Work out the finished part from the listing and answer in its coordinate system (mm). A direction names the side the tool comes from. Round coordinates to 2 decimals unless told otherwise and drop trailing zeros. Order: outer loops, then holes, each group sorted by start corner. A loop starts at its lowest first (then second) coordinate and runs counter-clockwise, first axis right, second up. Notation, with made-up numbers: (-30, 19.25) - (-15, 19.25) arc R10 cw to (-15, 38.25) - close; hole circle Ø2 at (49.5, 71). An arc over 180 degrees is marked (long way). Answer in a Markdown table with one row per item.
from build123d import *

# Parameters (mm, degrees)
SKETCH8_W           = 131.76
SKETCH8_H           = 95.69
SKETCH8_R           = 3.43
SKETCH8_W_2         = 73.4
SKETCH8_H_2         = 33.99
BOSS_EXTRUDE4_DEPTH = 40
SKETCH9_R           = 8
CUT_EXTRUDE2_DEPTH  = 8
SKETCH12_W          = 9.12
SKETCH12_H          = 95.69
BOSS_EXTRUDE5_DEPTH = 40
SKETCH13_W          = 150
SKETCH13_H          = 50.05
BOSS_EXTRUDE6_DEPTH = 26.38
SKETCH14_R          = 3.05
CUT_EXTRUDE3_DEPTH  = 3.05


with BuildPart() as part:
    # Sketch8 → Boss-Extrude4 (new body)
    with BuildSketch(Plane(origin=(0, 0, 0), x_dir=(1, 0, 0), z_dir=(0, 1, 0))):
        with Locations((-55.88, 37.845)):
            Rectangle(SKETCH8_W, SKETCH8_H)
        with Locations((-100.58, 12.85)):
            Circle(SKETCH8_R, mode=Mode.SUBTRACT)
        with Locations((-100.58, 62.84)):
            Circle(SKETCH8_R, mode=Mode.SUBTRACT)
        with Locations((-11.18, 62.84)):
            Circle(SKETCH8_R, mode=Mode.SUBTRACT)
        with Locations((-11.18, 12.85)):
            Circle(SKETCH8_R, mode=Mode.SUBTRACT)
        with Locations((-55.88, 37.845)):
            Rectangle(SKETCH8_W_2, SKETCH8_H_2, mode=Mode.SUBTRACT)
    extrude(amount=BOSS_EXTRUDE4_DEPTH)

    # Sketch9 → Cut-Extrude2 (cut)
    with BuildSketch(Plane.XZ):
        with Locations((-100.58, -12.85)):
            Circle(SKETCH9_R)
        with Locations((-11.18, -12.85)):
            Circle(SKETCH9_R)
        with Locations((-11.18, -62.84)):
            Circle(SKETCH9_R)
        with Locations((-100.58, -62.84)):
            Circle(SKETCH9_R)
    extrude(amount=-CUT_EXTRUDE2_DEPTH, mode=Mode.SUBTRACT)

    # Sketch12 → Boss-Extrude5 (add)
    with BuildSketch(Plane.XZ):
        with Locations((-126.32, -37.845)):
            Rectangle(SKETCH12_W, SKETCH12_H)
        with Locations((14.56, -37.845)):
            Rectangle(SKETCH12_W, SKETCH12_H)
    extrude(amount=-BOSS_EXTRUDE5_DEPTH)

    # Sketch13 → Boss-Extrude6 (add)
    with BuildSketch(Plane.XZ):
        with Locations((-55.88, 35.025)):
            Rectangle(SKETCH13_W, SKETCH13_H)
    extrude(amount=-BOSS_EXTRUDE6_DEPTH)

    # Sketch14 → Cut-Extrude3 (cut)
    with BuildSketch(Plane(origin=(0, 26.38, 0), x_dir=(1, 0, 0), z_dir=(0, 1, 0))):
        with Locations((-105.88, -22.5125)):
            Circle(SKETCH14_R)
        with Locations((-105.88, -47.5375)):
            Circle(SKETCH14_R)
        with BuildLine():
            ThreePointArc((-77.83, -35.025), (-80.88, -31.975), (-83.93, -35.025))
            Line((-83.93, -35.025), (-77.83, -35.025))
        make_face()
        with BuildLine():
            Line((-77.83, -35.025), (-83.93, -35.025))
            ThreePointArc((-83.93, -35.025), (-80.88, -38.075), (-77.83, -35.025))
        make_face()
        with BuildLine():
            ThreePointArc((-52.83, -22.5125), (-53.723324317, -20.355824317), (-55.88, -19.4625))
            Line((-55.88, -19.4625), (-55.88, -25.5625))
            ThreePointArc((-55.88, -25.5625), (-53.723324317, -24.669175683), (-52.83, -22.5125))
        make_face()
        with BuildLine():
            Line((-55.88, -25.5625), (-55.88, -19.4625))
            ThreePointArc((-55.88, -19.4625), (-58.93, -22.5125), (-55.88, -25.5625))
        make_face()
        with BuildLine():
            ThreePointArc((-55.88, -44.4875), (-58.93, -47.5375), (-55.88, -50.5875))
            Line((-55.88, -50.5875), (-55.88, -44.4875))
        make_face()
        with BuildLine():
            Line((-55.88, -44.4875), (-55.88, -50.5875))
            ThreePointArc((-55.88, -50.5875), (-53.723324317, -49.694175683), (-52.83, -47.5375))
            ThreePointArc((-52.83, -47.5375), (-53.723324317, -45.380824317), (-55.88, -44.4875))
        make_face()
        with BuildLine():
            ThreePointArc((-33.93, -35.025), (-33.036675683, -37.181675683), (-30.88, -38.075))
            Line((-30.88, -38.075), (-30.88, -35.025))
            Line((-30.88, -35.025), (-33.93, -35.025))
        make_face()
        with BuildLine():
            Line((-30.88, -35.025), (-30.88, -38.075))
            ThreePointArc((-30.88, -38.075), (-28.723324317, -37.181675683), (-27.83, -35.025))
            Line((-27.83, -35.025), (-30.88, -35.025))
        make_face()
        with BuildLine():
            ThreePointArc((-27.83, -35.025), (-28.723324317, -32.868324317), (-30.88, -31.975))
            Line((-30.88, -31.975), (-30.88, -35.025))
            Line((-30.88, -35.025), (-27.83, -35.025))
        make_face()
        with BuildLine():
            Line((-30.88, -35.025), (-30.88, -31.975))
            ThreePointArc((-30.88, -31.975), (-33.036675683, -32.868324317), (-33.93, -35.025))
            Line((-33.93, -35.025), (-30.88, -35.025))
        make_face()
        with BuildLine():
            ThreePointArc((-2.83, -22.5125), (-3.723324317, -20.355824317), (-5.88, -19.4625))
            Line((-5.88, -19.4625), (-5.88, -25.5625))
            ThreePointArc((-5.88, -25.5625), (-3.723324317, -24.669175683), (-2.83, -22.5125))
        make_face()
        with BuildLine():
            Line((-5.88, -25.5625), (-5.88, -19.4625))
            ThreePointArc((-5.88, -19.4625), (-8.93, -22.5125), (-5.88, -25.5625))
        make_face()
        with BuildLine():
            ThreePointArc((-5.88, -44.4875), (-8.93, -47.5375), (-5.88, -50.5875))
            Line((-5.88, -50.5875), (-5.88, -44.4875))
        make_face()
        with BuildLine():
            Line((-5.88, -44.4875), (-5.88, -50.5875))
            ThreePointArc((-5.88, -50.5875), (-3.723324317, -49.694175683), (-2.83, -47.5375))
            ThreePointArc((-2.83, -47.5375), (-3.723324317, -45.380824317), (-5.88, -44.4875))
        make_face()
    extrude(amount=-CUT_EXTRUDE3_DEPTH, mode=Mode.SUBTRACT)


solid = part.part
1) The mould has two halves that part along X. Classify faces 1 (the face through (-57, 13, 60.05)), 2 (the face through (-6, 23.33, 22)): released by +X, released by -X, zero draft, split by the parting line, or undercut.
Filled in:
| item | result |
|---|---|
| face 1 | zero draft |
| face 2 | undercut |
2) Find section D-D, the plane z = -12.85. Give the vertices of the cut face in (x, y), then the cut area to 3 significant figures.
Filled in:
| item | result |
|---|---|
| outline | (-130.88, 0) - (-108.58, 0) - (-108.58, 8) - (-104.01, 8) - (-104.01, 40) - (-130.88, 40) - close; (-97.15, 8) - (-92.58, 8) - (-92.58, 0) - (-19.18, 0) - (-19.18, 8) - (-14.61, 8) - (-14.61, 40) - (-97.15, 40) - close; (-7.75, 8) - (-3.18, 8) - (-3.18, 0) - (19.12, 0) - (19.12, 40) - (-7.75, 40) - close |
| area | 5,300 mm^2 |
3) Find section A-A, the plane x = -80.88. Give the vertices of the cut face in (y, z) (3 decimals), then the cut area to 3 significant figures.
Filled in:
| item | result |
|---|---|
| outline | (0, -85.69) - (40, -85.69) - (40, -54.84) - (0, -54.84) - close; (0, -20.85) - (40, -20.85) - (40, 10) - (26.38, 10) - (26.38, 31.975) - (23.33, 31.975) - (23.33, 38.075) - (26.38, 38.075) - (26.38, 60.05) - (0, 60.05) - close |
| area | 3,770 mm^2 |
4) Find section B-B, the plane z = -47. Give the vertices of the cut face in (x, y), then the cut area to 3 significant figures.
Filled in:
| item | result |
|---|---|
| outline | (-130.88, 0) - (-92.58, 0) - (-92.58, 40) - (-130.88, 40) - close; (-19.18, 0) - (19.12, 0) - (19.12, 40) - (-19.18, 40) - close |
| area | 3,060 mm^2 |
5) Find the intervals of material crossed by probe 1 along Z at (x, y) = (-100.58, 4.5); probe 2 along X at (y, z) = (16, -62.84); probe 3 along Z at (x, y) = (-105.88, 25.75), in increasing order. Write a range as from..to.
Filled in:
| item | result |
|---|---|
| probe 1 | z = -85.69..-70.84, -54.84..-20.85, -4.85..60.05 |
| probe 2 | x = -130.88..-104.01, -97.15..-14.61, -7.75..19.12 |
| probe 3 | z = -85.69..19.46, 25.56..44.49, 50.59..60.05 |
6) Find section C-C, the plane x = -11.18. Give the vertices of the cut face in (y, z), then the cut area to 3 significant figures.
Filled in:
| item | result |
|---|---|
| outline | (0, -85.69) - (40, -85.69) - (40, -66.27) - (8, -66.27) - (8, -70.84) - (0, -70.84) - close; (0, -54.84) - (8, -54.84) - (8, -59.41) - (40, -59.41) - (40, -16.28) - (8, -16.28) - (8, -20.85) - (0, -20.85) - close; (0, -4.85) - (8, -4.85) - (8, -9.42) - (40, -9.42) - (40, 10) - (26.38, 10) - (26.38, 60.05) - (0, 60.05) - close |
| area | 4,450 mm^2 |
7) Which of the six approach directions +Z, -Z, +X, -X, +Y, -Y give full straight-line access (tool end or side, diameter ignored) to faces 3 (the face through (-19.18, 20, -38)), 4 (the face through (-9.5, 8, -16.3)), 5 (the face through (-57, 40, -16)), 6 (the face through (-57, 0, -12)), 7 (the face through (-77.833, 24.876, 35.159))?
Filled in:
| item | result |
|---|---|
| face 3 | +Y, -Y |
| face 4 | -Y |
| face 5 | +Z, -Z, +X, -X, +Y |
| face 6 | +Z, -Z, +X, -X, -Y |
| face 7 | +Y |
8) Each of these flat-tipped pins is pushed along its axis until it touches: pin 1 (1.8 mm diameter, centred on x = -5, z = 49, fed in from +Y); pin 2 (10 mm diameter, centred on x = -105.88, z = 22.51, fed in from +Y); pin 3 (14.5 mm diameter, centred on x = -11.18, z = -12.85, fed in from -Y). Where does it stop, or does it pass through?
Filled in:
| item | result |
|---|---|
| pin 1 | stops at y = 23.33 |
| pin 2 | stops at y = 26.38 |
| pin 3 | stops at y = 8 |
